Design review of the part built by this model. Coordinates are the model's own, in mm. Coordinates: 2 decimals unless noted, no trailing zeros. Loops run counter-clockwise (first coordinate to the right, second up) from the corner with the lowest first, then second, coordinate; pieces in that order, holes last. Notation, with made-up numbers: M 64.5,21.25 L 71.5,21.25 A22 ccw 71.5,55.25 Z; hole C 24.5,47.25 d6. An arc over 180 degrees is marked long. Answer as a JSON object with one key per item and string values. Group by question number.
1. Insertion check: pin 1 (3.5 mm diameter, centred on y = 106.5, z = -4, fed in from +X); pin 2 (1.5 mm diameter, centred on x = 2, z = 31.5, fed in from -Y); pin 3 (1.5 mm diameter, centred on x = 1.5, z = -0.5, fed in from +Y); pin 4 (2 mm diameter, centred on x = 2.5, z = 22, fed in from +Y). Each pin has a flat end and moves straight along its axis. Give the tip position at first contact, or say it passes through.
2. Consider section B-B (y = 85.75). State the section outline as (x, z) points, then the cut area to 3 significant figures.
3. Consider section A-A (y = 3). State the section outline as (x, z) points.
4. To check wall thickness, follow probe 1 along Y at (x, z) = (3.55, 15); probe 2 along Y at (x, z) = (1.55, 15); probe 3 along Y at (x, z) = (2.25, 11.5). State the ranges of each line that lie inside material, in increasing order.
5. Consider section D-D (z = 34.25). State the section outline as (x, y) points, then the cut area to 3 significant figures.
6. Consider section C-C (z = 10.5). State the section outline as (x, y) points, then the cut area to 3 significant figures.
from build123d import *

# Parameters (mm, degrees)
SKETCH_1_W                  = 5
SKETCH_1_H                  = 30
EXTRUDE_1_DEPTH             = 227
SKETCH_2_R                  = 22.5
EXTRUDE_2_DEPTH             = 5
SKETCH_3_R                  = 14
CUT_EXTRUDE_1_DEPTH         = 231.130940988
HOLE_WIZARD_M31_D           = 3.4
HOLE_WIZARD_M31_CBORE_D     = 6.7
HOLE_WIZARD_M31_CBORE_DEPTH = 2
EXTRUDE_3_DEPTH             = 5
HOLE_WIZARD_M31_2_D         = 3.4
SKETCH_14_W                 = 45
SKETCH_14_H                 = 6
CUT_EXTRUDE_2_DEPTH         = 1
CUT_EXTRUDE_START           = -5
CUT_EXTRUDE_3_DEPTH         = 5


with BuildPart() as part:
    # Эскиз1 → Бобышка-Вытянуть1 (new body)
    with BuildSketch(Plane(origin=(0, 0, 0), x_dir=(1, 0, 0), z_dir=(0, 1, 0))):
        with Locations((2.5, -15)):
            Rectangle(SKETCH_1_W, SKETCH_1_H)
    extrude(amount=EXTRUDE_1_DEPTH)

    # Эскиз2 → Бобышка-Вытянуть2 (add)
    with BuildSketch(Plane.ZY):
        with Locations((15, 105)):
            Circle(SKETCH_2_R)
    extrude(amount=-EXTRUDE_2_DEPTH)

    # Эскиз3 → Вырез-Вытянуть1 (cut, through all)
    with BuildSketch(Plane.ZY):
        with Locations((15, 105)):
            Circle(SKETCH_3_R)
    extrude(amount=-CUT_EXTRUDE_1_DEPTH, mode=Mode.SUBTRACT)

    # Hole Wizard M31 (through all)
    with Locations(Plane(origin=(5, -25.024735225, 7.262908886), x_dir=(0, 0, 1), z_dir=(1, 0, 0))):
        with Locations((7.737091114, -149.274735225), (-11.512908886, -130.024735225), (7.737091114, -110.774735225), (26.987091114, -130.024735225)):
            CounterBoreHole(HOLE_WIZARD_M31_D / 2, HOLE_WIZARD_M31_CBORE_D / 2, HOLE_WIZARD_M31_CBORE_DEPTH)

    # Эскиз11 → Бобышка-Вытянуть3 (add)
    with BuildSketch(Plane(origin=(5, 0, 0), x_dir=(0, 0, -1), z_dir=(1, 0, 0))):
        Polygon((0, 18.990381057), (7.5, 6), (7.5, 0), (-37.5, 0), (-37.5, 6), (-30, 18.990381057), align=None)
    extrude(amount=-EXTRUDE_3_DEPTH)

    # Hole Wizard M31 2 (through all)
    with Locations(Plane(origin=(5, 0, 0), x_dir=(0, 0, -1), z_dir=(1, 0, 0))):
        with Locations((-28.5, 3), (-19.5, 3), (-10.5, 3), (-1.5, 3)):
            Hole(HOLE_WIZARD_M31_2_D / 2)

    # Эскиз14 → Вырез-Вытянуть2 (cut)
    with BuildSketch(Plane(origin=(5, 0, 0), x_dir=(0, 0, -1), z_dir=(1, 0, 0))):
        with Locations((-15, 3)):
            Rectangle(SKETCH_14_W, SKETCH_14_H)
    extrude(amount=-CUT_EXTRUDE_2_DEPTH, mode=Mode.SUBTRACT)

    # Эскиз15 → Вырез-Вытянуть3 (cut)
    with BuildSketch(Plane(origin=(5, 0, 0), x_dir=(0, 0, -1), z_dir=(1, 0, 0)).offset(CUT_EXTRUDE_START)):
        with BuildLine():
            Line((-30, 227), (0, 227))
            Line((0, 227), (0, 121.770509831))
            ThreePointArc((0, 121.770509831), (-15, 127.5), (-30, 121.770509831))
            Line((-30, 121.770509831), (-30, 227))
        make_face()
    extrude(amount=CUT_EXTRUDE_3_DEPTH, mode=Mode.SUBTRACT)


solid = part.part
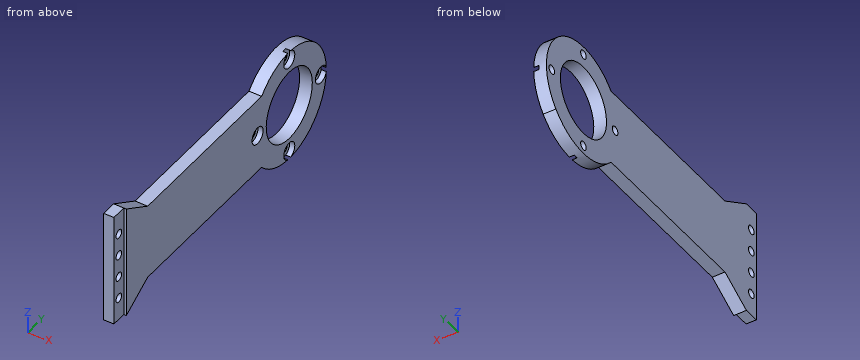
Findings below:
{
 "1": {"pin 1": "stops at x = 3", "pin 2": "stops at y = 0", "pin 3": "stops at y = 121.99", "pin 4": "stops at y = 126.69"},
 "2": {"outline": "M 0,0 L 5,0 L 5,11.65 L 3,11.65 L 3,13.3 L 0,13.3 Z; M 0,16.7 L 3,16.7 L 3,18.35 L 5,18.35 L 5,30 L 0,30 Z", "area": "126 mm^2"},
 "3": {"outline": "M 0,-7.5 L 4,-7.5 L 4,-0.2 L 0,-0.2 Z; M 0,3.2 L 4,3.2 L 4,8.8 L 0,8.8 Z; M 0,12.2 L 4,12.2 L 4,17.8 L 0,17.8 Z; M 0,21.2 L 4,21.2 L 4,26.8 L 0,26.8 Z; M 0,30.2 L 4,30.2 L 4,37.5 L 0,37.5 Z"},
 "4": {"probe 1": "y = 0 to 82.4, 89.1 to 91, 119 to 120.9", "probe 2": "y = 0 to 84.05, 87.45 to 91, 119 to 122.55, 125.95 to 127.5", "probe 3": "y = 0 to 1.63, 4.37 to 91.44, 118.56 to 127.23"},
 "5": {"outline": "M 0,0 L 4,0 L 4,6 L 5,6 L 5,11.63 L 0,11.63 Z; M 0,93.35 L 5,93.35 L 5,101.65 L 3,101.65 L 3,103.3 L 0,103.3 Z; M 0,106.7 L 3,106.7 L 3,108.35 L 5,108.35 L 5,116.65 L 0,116.65 Z", "area": "145 mm^2"},
 "6": {"outline": "M 0,0 L 4,0 L 4,1.3 L 0,1.3 Z; M 0,4.7 L 4,4.7 L 4,6 L 5,6 L 5,91.74 L 0,91.74 Z; M 0,118.26 L 5,118.26 L 5,127.05 L 0,127.05 Z", "area": "483 mm^2"}
}
